Verification items for this drawing (mm, ordinates from the low corner). Round coordinates to 2 decimals unless told otherwise and drop trailing zeros. Loops run counter-clockwise (first coordinate to the right, second up) from the corner with the lowest first, then second, coordinate; pieces in that order, holes last. Notation, with made-up numbers: (78, 13) - (131, 13) arc R21 ccw to (131, 43) - close; hole circle Ø5 at (-20, 16). An arc over 180 degrees is marked (long way). Put each result on its own line as item: value.
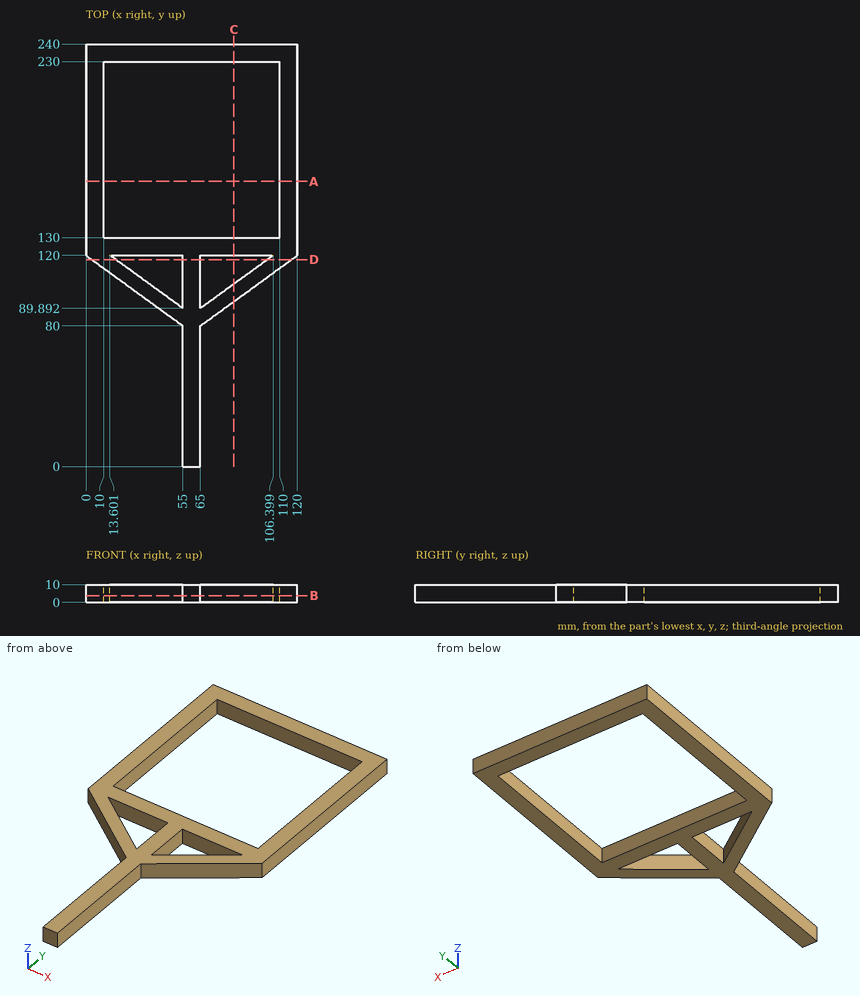
Item 1: Section check D-D on y = 117.5. Enter the section's corners in (x, z).
Filled sheet:
outline: (3.44, 0) - (17.04, 0) - (17.04, 10) - (3.44, 10) - close; (55, 0) - (65, 0) - (65, 10) - (55, 10) - close; (102.96, 0) - (116.56, 0) - (116.56, 10) - (102.96, 10) - close
Item 2: Thickness scan on line 1 (Y direction, x = 40, z = 3.5); line 2 (Y direction, x = 31.5, z = 4) (1 decimal); line 3 (X direction, y = 203, z = 5). Record the ranges inside material, lowest first. Write a range as from..to.
Filled sheet:
line 1: 90.91..100.8, 120..130, 230..240
line 2: 97.1..107, 120..130, 230..240
line 3: 0..10, 110..120
Item 3: Section check C-C on x = 84. Enter the section's corners in (y, z).
Filled sheet:
outline: (93.82, 0) - (103.71, 0) - (103.71, 10) - (93.82, 10) - close; (120, 0) - (130, 0) - (130, 10) - (120, 10) - close; (230, 0) - (240, 0) - (240, 10) - (230, 10) - close
Item 4: Section check A-A on y = 162. Enter the section's corners in (x, z).
Filled sheet:
outline: (0, 0) - (10, 0) - (10, 10) - (0, 10) - close; (110, 0) - (120, 0) - (120, 10) - (110, 10) - close
Item 5: Section check B-B on z = 3.75. Enter the section's corners in (x, y).
Filled sheet:
outline: (0, 120) - (55, 80) - (55, 0) - (65, 0) - (65, 80) - (120, 120) - (120, 240) - (0, 240) - close; hole (10, 130) - (110, 130) - (110, 230) - (10, 230) - close; hole (13.6, 120) - (55, 89.89) - (55, 120) - close; hole (65, 89.89) - (106.4, 120) - (65, 120) - close
Item 6: Go/stop test with flat-tipped pins: pin 1 (4 mm diameter, centred on x = 27.5, z = 5.5, fed in from -Y) (1 decimal); pin 2 (1.5 mm diameter, centred on x = 103.5, z = 4, fed in from -Y) (1 decimal); pin 3 (1 mm diameter, centred on y = 56, z = 1.5, fed in from +X); pin 4 (8 mm diameter, centred on x = 103.5, y = 181.5, fed in from +Z). Record where each tip stops, or that it passes through.
Filled sheet:
pin 1: y = 98.5
pin 2: y = 107.5
pin 3: x = 65
pin 4: through
